For this review, take the finished solid that the model builds, in its own axes (mm). Coordinates: 2 decimals unless noted, no trailing zeros. Order: outer loops, then holes, each group sorted by start corner. A loop starts at its lowest first (then second) coordinate and runs counter-clockwise, first axis right, second up. Notation, with made-up numbers: (55, 59.25) -> (104, 59.25) arc R32 cw to (104, 96.25) -> close; hole circle Ø6 at (-39, -14). An arc over 180 degrees is marked (long way). Answer as a JSON object with one key per item and string values. Group by question number.
1) Add section B-B, the plane x = 0. Write out the cut boundary in (y, z), then the cut area to 3 significant figures.
2) Add section A-A, the plane z = 0. Write out the cut boundary in (x, y), then the cut area to 3 significant figures.
3) For pin 1 (3 mm diameter, centred on x = 2.5, z = -1.5, fed in from -Y); pin 2 (1.5 mm diameter, centred on y = 151.5, z = -2, fed in from +X); pin 3 (1.5 mm diameter, centred on x = 1.5, z = 3.5, fed in from -Y); pin 4 (5 mm diameter, centred on x = -3.5, y = 75.5, fed in from -Z), all flat-tipped, find the tip position at first contact; note any pin that passes through.
4) Add section C-C, the plane y = 139.5. Write out the cut boundary in (x, z), then the cut area to 3 significant figures.
5) Wall thickness on L1, parallel to Z at x = 0, y = 83.5; L2, parallel to Z at x = -1, y = 54; L3, parallel to X at y = 50.5, z = -0.75: over which ranges is each line inside the solid? List them lowest first.
from build123d import *

# Parameters (mm, degrees)
F0_R     = 4.7
F0_R_2   = 4.5
F1_DEPTH = 200


with BuildPart() as f1:
    # F0 (on Front) → F1 (new body)
    with BuildSketch(Plane.XZ):
        Circle(F0_R)
        Circle(F0_R_2, mode=Mode.SUBTRACT)
    extrude(amount=-F1_DEPTH)


with BuildPart() as f3_1:
    # F3: instance of F1
    add(f1.part.mirror(Plane.YZ.offset(-15)))


solid = f1.part
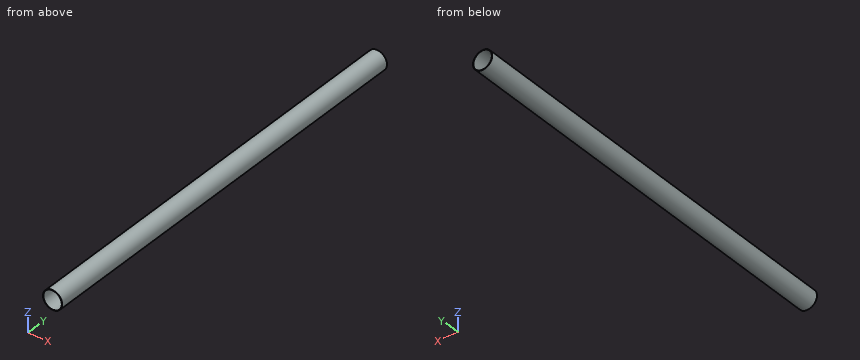
Output values:
{
 "1": {"outline": "(0, -4.7) -> (200, -4.7) -> (200, -4.5) -> (0, -4.5) -> close; (0, 4.5) -> (200, 4.5) -> (200, 4.7) -> (0, 4.7) -> close", "area": "80.0 mm²"},
 "2": {"outline": "(-4.7, 0) -> (-4.5, 0) -> (-4.5, 200) -> (-4.7, 200) -> close; (4.5, 0) -> (4.7, 0) -> (4.7, 200) -> (4.5, 200) -> close", "area": "80.0 mm²"},
 "3": {"pin 1": "passes through", "pin 2": "stops at x = 4.53", "pin 3": "stops at y = 0", "pin 4": "stops at z = -4.59"},
 "4": {"outline": "circle Ø9.4 at (0, 0); hole circle Ø9 at (0, 0)", "area": "5.78 mm²"},
 "5": {"L1": "z = -4.7 to -4.5, 4.5 to 4.7", "L2": "z = -4.59 to -4.39, 4.39 to 4.59", "L3": "x = -4.64 to -4.44, 4.44 to 4.64"}
}
